Could you check a few things on this model? Use its own coordinates, in mm. A direction names the side the tool comes from. Give positions to 0.01 mm unless a question says otherwise; leave off trailing zeros. Order: outer loops, then holes, each group sorted by start corner. A loop starts at its lowest first (then second) coordinate and runs counter-clockwise, first axis right, second up.
from build123d import *

# Parameters (mm, degrees)
SALIENTE_EXTRUIR1_DEPTH      = 3
SALIENTE_EXTRUIR2_DEPTH      = 9
SALIENTE_EXTRUIR3_DEPTH      = 24
CORTAR_EXTRUIR1_DEPTH        = 3
CORTAR_EXTRUIR_L_MINA1_START = -2.993325909
CORTAR_EXTRUIR_L_MINA1_DEPTH = 2.993325909
REDONDEO1_R                  = 2
CROQUIS6_R                   = 1.25
CORTAR_EXTRUIR2_DEPTH        = 3
CROQUIS7_R                   = 1.5
CORTAR_EXTRUIR3_DEPTH        = 3


# Read off the part's stored shape, not the designer's step: Cortar-Extruir-Lámina1
with BuildPart() as part:
    # Croquis1 → Saliente-Extruir1 (new body)
    with BuildSketch(Plane.XY):
        Polygon((0, 0), (20, 0), (22, 29.933259094), (-2, 29.933259094), align=None)
    extrude(amount=SALIENTE_EXTRUIR1_DEPTH)

    # Croquis2 → Saliente-Extruir2 (add)
    with BuildSketch(Plane.XY.offset(3)):
        Polygon((0, 0), (20, 0), (20.2, 2.993325909), (-0.2, 2.993325909), align=None)
    extrude(amount=SALIENTE_EXTRUIR2_DEPTH)

    # Croquis3 → Saliente-Extruir3 (add)
    with BuildSketch(Plane.XY.offset(3)):
        Polygon((22, 29.933259094), (21.8, 26.939933185), (-1.8, 26.939933185), (-2, 29.933259094), align=None)
    extrude(amount=SALIENTE_EXTRUIR3_DEPTH)

    # Croquis4 → Cortar-Extruir1 (cut)
    with BuildSketch(Plane.XY.offset(3)):
        with BuildLine():
            Line((17.5, 26.939933185), (17.5, 23.939933185))
            ThreePointArc((17.5, 23.939933185), (10, 16.499759469), (2.5, 23.939933185))
            Line((2.5, 23.939933185), (2.5, 26.939933185))
            Line((2.5, 26.939933185), (17.5, 26.939933185))
        make_face()
    extrude(amount=-CORTAR_EXTRUIR1_DEPTH, mode=Mode.SUBTRACT)

    # Cortar-Extruir-Lámina1 outline → Cortar-Extruir-Lámina1 (cut)
    with BuildSketch(Plane.XZ.offset(-26.939933185).offset(CORTAR_EXTRUIR_L_MINA1_START)):
        with BuildLine():
            Line((2.5, 0), (17.5, 0))
            Line((17.5, 0), (17.5, 3))
            ThreePointArc((17.5, 3), (10, 10.5), (2.5, 3))
            Line((2.5, 3), (2.5, 0))
        make_face()
    extrude(amount=CORTAR_EXTRUIR_L_MINA1_DEPTH, mode=Mode.SUBTRACT)

    # Redondeo1
    redondeo1_edges = [part.edges().sort_by_distance(p)[0] for p in [
        (-0.1, 1.496662955, 12),
        (20.1, 1.496662955, 12),
        (-1.9, 28.436596139, 27),
        (21.9, 28.436596139, 27),
        (19.75, 29.933259094, 0),
        (0.25, 29.933259094, 0),
    ]]
    fillet(redondeo1_edges, radius=REDONDEO1_R)

    # Croquis6 → Cortar-Extruir2 (cut)
    with BuildSketch(Plane.XZ.offset(-26.939933185)):
        with Locations((10, 20)):
            Circle(CROQUIS6_R)
    extrude(amount=-CORTAR_EXTRUIR2_DEPTH, mode=Mode.SUBTRACT)

    # Croquis7 → Cortar-Extruir3 (cut)
    with BuildSketch(Plane.XZ):
        with Locations(Location((4, 6.5, 0), (0, 0, 270))):
            Circle(CROQUIS7_R)
        with Locations((16, 6.5)):
            Circle(CROQUIS7_R)
    extrude(amount=-CORTAR_EXTRUIR3_DEPTH, mode=Mode.SUBTRACT)


solid = part.part
Item 1: Imagine slicing it at B-B on y = 25.5. List the corners of the cut face in (x, z) for me, then the cut area to 3 significant figures.
Findings:
outline: (-1.7, 0) - (2.5, 0) - (2.5, 3) - (-1.7, 3) - close; (17.5, 0) - (21.7, 0) - (21.7, 3) - (17.5, 3) - close
area: 25.2 mm2
Item 2: Imagine slicing it at A-A on x = 10. List the corners of the cut face in (y, z) for me.
Findings:
outline: (0, 0) - (16.5, 0) - (16.5, 3) - (2.99, 3) - (2.99, 12) - (0, 12) - close; (26.94, 10.5) - (29.93, 10.5) - (29.93, 18.75) - (26.94, 18.75) - close; (26.94, 21.25) - (29.93, 21.25) - (29.93, 27) - (26.94, 27) - close
Item 3: Imagine slicing it at D-D on x = 7.5. List the corners of the cut face in (y, z) for me, then the cut area to 3 significant figures.
Findings:
outline: (0, 0) - (16.93, 0) - (16.93, 3) - (2.99, 3) - (2.99, 12) - (0, 12) - close; (26.94, 10.07) - (29.93, 10.07) - (29.93, 27) - (26.94, 27) - close
area: 128 mm2
Item 4: For faces 4 (the flat face through (17.5, 27, 1)), 5 (the cylindrical face through (0.22, 29.33, 0.57)), 6 (the flat face through (10, 12, 3)), 7 (the flat face through (10, 2, 12)), 8 (the cylindrical face through (4, 1, 8)), which set-ups out of +Z, -Z, +X, -X, +Y, -Y let a thin tool reach every point of the face, with its end or its side?
Findings:
face 4: -Z, +Y
face 5: -Z, +X, -X, +Y
face 6: +Z, +X, -X
face 7: +Z, +X, -X, -Y
face 8: -Y
Item 5: For pin 1 (8 mm diameter, centred on x = 10.5, y = 16.5, fed in from +Z); pin 2 (0.9 mm diameter, centred on y = 28, z = 2, fed in from +X); pin 3 (0.9 mm diameter, centred on x = 6.5, y = 1, fed in from +Z), each with a flat end and sliding along its axis, tell me the tip position at first contact or that it passes through.
Findings:
pin 1: stops at z = 3
pin 2: stops at x = 21.9
pin 3: stops at z = 12
Item 6: Imagine slicing it at C-C on z = 11. List the corners of the cut face in (x, y) for me, then the cut area to 3 significant figures.
Findings:
outline: (-2, 29.93) - (-1.8, 26.94) - (21.8, 26.94) - (22, 29.93) - close; (0.07, 2.99) - (0.27, 0) - (19.73, 0) - (19.93, 2.99) - close
area: 130 mm2
Item 7: We'd pull the mould along Z, two halves only. Please class faces 1 (the flat face through (10, 28, 27)), 2 (the cylindrical face through (10.16, 28.46, 10.5)), 3 (the cylindrical face through (9.01, 28.42, 19.24)): +Z half, -Z half, draft (parallel to the pull), parting line (faces both ways), or undercut.
Findings:
face 1: +Z half
face 2: -Z half
face 3: undercut
Item 8: Please list where these lines run through material, in increasing order: line 1 along Z through (x, y) = (16, 1.25); line 2 along Y through (x, z) = (0.75, 7); line 3 along X through (y, z) = (19, 1).
Findings:
line 1: z = 0 to 5, 8 to 12
line 2: y = 0 to 2.99, 26.94 to 29.93
line 3: x = -1.27 to 4.41, 15.59 to 21.27
